Source: CAD feature listing. Evaluate the final solid. Frame: model axes, mm. A direction names the side the tool comes from. Round coordinates to 2 decimals unless told otherwise and drop trailing zeros. Order: outer loops, then holes, each group sorted by start corner. A loop starts at its lowest first (then second) coordinate and runs counter-clockwise, first axis right, second up. Notation, with made-up numbers: (6.5, 6.5) - (62.5, 6.5) arc R18 cw to (62.5, 13.5) - close; hole circle Ø10 at (33, 72.25). An arc over 180 degrees is marked (long way). Return JSON: item names as keys, results as strings. Group by question number.
1) Section A-A, the plane y = 8. Return loops of the section in (x, z).
2) Mould query, pull axis Z, two halves, no side actions, for faces 1 (the flat face through (4, 12.223, 7)), 2 (the cylindrical face through (-13.7, -10.8, 14.4)), 3 (the cylindrical face through (25.8, 9.7, 8)). Classes: pulls with the +Z half, pulls with the -Z half, needs draft (parallel to the pull), parting line crosses it, or undercut.
3) Ray query, line 1 (Y direction, x = -5, z = 4); line 2 (X direction, y = -20, z = 3); line 3 (Y direction, x = 25, z = 12.5). Return the intervals inside material, ascending. Write a range as from..to.
4) Section D-D, the plane y = -4.5. Return loops of the section in (x, z), plus the area to 3 significant figures.
5) Access query for faces 4 (the cylindrical face through (20.126, -8.102, 0.57)), 5 (the flat face through (3, -20.777, 4)), 6 (the cylindrical face through (20.126, -10.36, 14.43)), 7 (the cylindrical face through (22.13, 5.7, 9.43)). Directions: +Z, -Z, +X, -X, +Y, -Y. A direction counts if a zero-diameter tool reaches every point of the face in a straight line with its end or side. Return the directions, or none.
6) Contact query for flat-ended pins moving along their axis: P1, Ø8, axis at y = -8, z = 10, coming from the +X side; P2, Ø2.5, axis at x = 24.23, z = 7.5, coming from the +Y side; P3, Ø4, axis at y = -12.5, z = 5, coming from the -X side. Output: stop coordinate, or through.
7) Section C-C, the plane z = 7.5. Give the number of separate pieces and of enclosed holes in the cut face, plus the area to 3 significant figures.
8) Section B-B, the plane x = 25. Return loops of the section in (y, z).
```python
from build123d import *

# Parameters (mm, degrees)
F0_W     = 35
F0_H     = 25
F0_H_2   = 1.58
F0_H_3   = 5
F1_DEPTH = 15
F3_DEPTH = 9
F4_R     = 2
F6_SIZE  = 2
F5_R     = 1.65
F7_R     = 1.65
F8_DEPTH = 8.0000008897
F5_R_2   = 2.85
F7_R_2   = 2.85
F9_DEPTH = 3


with BuildPart() as f1:
    # F0 (on Top) → F1 (new body)
    with BuildSketch(Plane.XY):
        Polygon((28.2275901735, 12.2229893546), (-21.7724098265, 12.2229893546), (-21.7724098265, 4.2229884648), (-14.2724098265, 4.2229884648), (20.7275901735, 4.2229884648), (28.2275901735, 4.2229884648), align=None)
        with Locations((3.2275901735, -8.2770115352)):
            Rectangle(F0_W, F0_H)
        with Locations((3.2275901735, -21.5670115352)):
            Rectangle(F0_W, F0_H_2)
        with Locations((3.2275901735, -24.8570115352)):
            Rectangle(F0_W, F0_H_3)
    extrude(amount=F1_DEPTH)

    # F2 (on face) → F3 (cut)
    with BuildSketch(Plane.XY):
        with BuildLine():
            Line((19.5775901735, -21.6070115352), (19.8775901735, -21.6070115352))
            ThreePointArc((19.8775901735, -21.6070115352), (20.195788225, -21.7388134836), (20.3275901735, -22.0570115352))
            Line((20.3275901735, -22.0570115352), (20.3275901735, -22.3570115352))
            Line((20.3275901735, -22.3570115352), (20.7275901735, -22.3570115352))
            Line((20.7275901735, -22.3570115352), (20.7275901735, -20.7770115352))
            Line((20.7275901735, -20.7770115352), (-14.2724098265, -20.7770115352))
            Line((-14.2724098265, -20.7770115352), (-14.2724098265, -22.3570115352))
            Line((-14.2724098265, -22.3570115352), (-14.1524098265, -22.3570115352))
            Line((-14.1524098265, -22.3570115352), (-14.1524098265, -22.0570115352))
            ThreePointArc((-14.1524098265, -22.0570115352), (-14.0206078781, -21.7388134836), (-13.7024098265, -21.6070115352))
            Line((-13.7024098265, -21.6070115352), (-13.6128300801, -21.6070115352))
            Line((-13.6128300801, -21.6070115352), (-13.4024098265, -21.6070115352))
            ThreePointArc((-13.4024098265, -21.6070115352), (-13.084211775, -21.7388134836), (-12.9524098265, -22.0570115352))
            Line((-12.9524098265, -22.0570115352), (-12.9524098265, -22.3570115352))
            Line((-12.9524098265, -22.3570115352), (-12.0724098265, -22.3570115352))
            Line((-12.0724098265, -22.3570115352), (-12.0724098265, -22.0570115352))
            ThreePointArc((-12.0724098265, -22.0570115352), (-11.9406078781, -21.7388134836), (-11.6224098265, -21.6070115352))
            Line((-11.6224098265, -21.6070115352), (-11.3224098265, -21.6070115352))
            ThreePointArc((-11.3224098265, -21.6070115352), (-11.004211775, -21.7388134836), (-10.8724098265, -22.0570115352))
            Line((-10.8724098265, -22.0570115352), (-10.8724098265, -22.3570115352))
            Line((-10.8724098265, -22.3570115352), (-9.9924098265, -22.3570115352))
            Line((-9.9924098265, -22.3570115352), (-9.9924098265, -22.0570115352))
            ThreePointArc((-9.9924098265, -22.0570115352), (-9.8606078781, -21.7388134836), (-9.5424098265, -21.6070115352))
            Line((-9.5424098265, -21.6070115352), (-9.2424098265, -21.6070115352))
            ThreePointArc((-9.2424098265, -21.6070115352), (-8.924211775, -21.7388134836), (-8.7924098265, -22.0570115352))
            Line((-8.7924098265, -22.0570115352), (-8.7924098265, -22.3570115352))
            Line((-8.7924098265, -22.3570115352), (-7.9124098265, -22.3570115352))
            Line((-7.9124098265, -22.3570115352), (-7.9124098265, -22.0570115352))
            ThreePointArc((-7.9124098265, -22.0570115352), (-7.7806078781, -21.7388134836), (-7.4624098265, -21.6070115352))
            Line((-7.4624098265, -21.6070115352), (-7.1624098265, -21.6070115352))
            ThreePointArc((-7.1624098265, -21.6070115352), (-6.844211775, -21.7388134836), (-6.7124098265, -22.0570115352))
            Line((-6.7124098265, -22.0570115352), (-6.7124098265, -22.3570115352))
            Line((-6.7124098265, -22.3570115352), (-5.8324098265, -22.3570115352))
            Line((-5.8324098265, -22.3570115352), (-5.8324098265, -22.0570115352))
            ThreePointArc((-5.8324098265, -22.0570115352), (-5.7006078781, -21.7388134836), (-5.3824098265, -21.6070115352))
            Line((-5.3824098265, -21.6070115352), (-5.0824098265, -21.6070115352))
            ThreePointArc((-5.0824098265, -21.6070115352), (-4.764211775, -21.7388134836), (-4.6324098265, -22.0570115352))
            Line((-4.6324098265, -22.0570115352), (-4.6324098265, -22.3570115352))
            Line((-4.6324098265, -22.3570115352), (-3.7524098265, -22.3570115352))
            Line((-3.7524098265, -22.3570115352), (-3.7524098265, -22.0570115352))
            ThreePointArc((-3.7524098265, -22.0570115352), (-3.6206078781, -21.7388134836), (-3.3024098265, -21.6070115352))
            Line((-3.3024098265, -21.6070115352), (-3.0024098265, -21.6070115352))
            ThreePointArc((-3.0024098265, -21.6070115352), (-2.684211775, -21.7388134836), (-2.5524098265, -22.0570115352))
            Line((-2.5524098265, -22.0570115352), (-2.5524098265, -22.3570115352))
            Line((-2.5524098265, -22.3570115352), (-1.6724098265, -22.3570115352))
            Line((-1.6724098265, -22.3570115352), (-1.6724098265, -22.0570115352))
            ThreePointArc((-1.6724098265, -22.0570115352), (-1.5406078781, -21.7388134836), (-1.2224098265, -21.6070115352))
            Line((-1.2224098265, -21.6070115352), (-0.9224098265, -21.6070115352))
            ThreePointArc((-0.9224098265, -21.6070115352), (-0.604211775, -21.7388134836), (-0.4724098265, -22.0570115352))
            Line((-0.4724098265, -22.0570115352), (-0.4724098265, -22.3570115352))
            Line((-0.4724098265, -22.3570115352), (0.4075901735, -22.3570115352))
            Line((0.4075901735, -22.3570115352), (0.4075901735, -22.0570115352))
            ThreePointArc((0.4075901735, -22.0570115352), (0.5393921219, -21.7388134836), (0.8575901735, -21.6070115352))
            Line((0.8575901735, -21.6070115352), (1.1575901735, -21.6070115352))
            ThreePointArc((1.1575901735, -21.6070115352), (1.475788225, -21.7388134836), (1.6075901735, -22.0570115352))
            Line((1.6075901735, -22.0570115352), (1.6075901735, -22.3570115352))
            Line((1.6075901735, -22.3570115352), (2.4875901735, -22.3570115352))
            Line((2.4875901735, -22.3570115352), (2.4875901735, -22.0570115352))
            ThreePointArc((2.4875901735, -22.0570115352), (2.6193921219, -21.7388134836), (2.9375901735, -21.6070115352))
            Line((2.9375901735, -21.6070115352), (3.2375901735, -21.6070115352))
            ThreePointArc((3.2375901735, -21.6070115352), (3.555788225, -21.7388134836), (3.6875901735, -22.0570115352))
            Line((3.6875901735, -22.0570115352), (3.6875901735, -22.3570115352))
            Line((3.6875901735, -22.3570115352), (4.5675901735, -22.3570115352))
            Line((4.5675901735, -22.3570115352), (4.5675901735, -22.0570115352))
            ThreePointArc((4.5675901735, -22.0570115352), (4.6993921219, -21.7388134836), (5.0175901735, -21.6070115352))
            Line((5.0175901735, -21.6070115352), (5.3175901735, -21.6070115352))
            ThreePointArc((5.3175901735, -21.6070115352), (5.635788225, -21.7388134836), (5.7675901735, -22.0570115352))
            Line((5.7675901735, -22.0570115352), (5.7675901735, -22.3570115352))
            Line((5.7675901735, -22.3570115352), (6.6475901735, -22.3570115352))
            Line((6.6475901735, -22.3570115352), (6.6475901735, -22.0570115352))
            ThreePointArc((6.6475901735, -22.0570115352), (6.7793921219, -21.7388134836), (7.0975901735, -21.6070115352))
            Line((7.0975901735, -21.6070115352), (7.3975901735, -21.6070115352))
            ThreePointArc((7.3975901735, -21.6070115352), (7.715788225, -21.7388134836), (7.8475901735, -22.0570115352))
            Line((7.8475901735, -22.0570115352), (7.8475901735, -22.3570115352))
            Line((7.8475901735, -22.3570115352), (8.7275901735, -22.3570115352))
            Line((8.7275901735, -22.3570115352), (8.7275901735, -22.0570115352))
            ThreePointArc((8.7275901735, -22.0570115352), (8.8593921219, -21.7388134836), (9.1775901735, -21.6070115352))
            Line((9.1775901735, -21.6070115352), (9.4775901735, -21.6070115352))
            ThreePointArc((9.4775901735, -21.6070115352), (9.795788225, -21.7388134836), (9.9275901735, -22.0570115352))
            Line((9.9275901735, -22.0570115352), (9.9275901735, -22.3570115352))
            Line((9.9275901735, -22.3570115352), (10.8075901735, -22.3570115352))
            Line((10.8075901735, -22.3570115352), (10.8075901735, -22.0570115352))
            ThreePointArc((10.8075901735, -22.0570115352), (10.9393921219, -21.7388134836), (11.2575901735, -21.6070115352))
            Line((11.2575901735, -21.6070115352), (11.5575901735, -21.6070115352))
            ThreePointArc((11.5575901735, -21.6070115352), (11.875788225, -21.7388134836), (12.0075901735, -22.0570115352))
            Line((12.0075901735, -22.0570115352), (12.0075901735, -22.3570115352))
            Line((12.0075901735, -22.3570115352), (12.8875901735, -22.3570115352))
            Line((12.8875901735, -22.3570115352), (12.8875901735, -22.0570115352))
            ThreePointArc((12.8875901735, -22.0570115352), (13.0193921219, -21.7388134836), (13.3375901735, -21.6070115352))
            Line((13.3375901735, -21.6070115352), (13.6375901735, -21.6070115352))
            ThreePointArc((13.6375901735, -21.6070115352), (13.955788225, -21.7388134836), (14.0875901735, -22.0570115352))
            Line((14.0875901735, -22.0570115352), (14.0875901735, -22.3570115352))
            Line((14.0875901735, -22.3570115352), (14.9675901735, -22.3570115352))
            Line((14.9675901735, -22.3570115352), (14.9675901735, -22.0570115352))
            ThreePointArc((14.9675901735, -22.0570115352), (15.0993921219, -21.7388134836), (15.4175901735, -21.6070115352))
            Line((15.4175901735, -21.6070115352), (15.7175901735, -21.6070115352))
            ThreePointArc((15.7175901735, -21.6070115352), (16.035788225, -21.7388134836), (16.1675901735, -22.0570115352))
            Line((16.1675901735, -22.0570115352), (16.1675901735, -22.3570115352))
            Line((16.1675901735, -22.3570115352), (17.0475901735, -22.3570115352))
            Line((17.0475901735, -22.3570115352), (17.0475901735, -22.0570115352))
            ThreePointArc((17.0475901735, -22.0570115352), (17.1793921219, -21.7388134836), (17.4975901735, -21.6070115352))
            Line((17.4975901735, -21.6070115352), (17.7975901735, -21.6070115352))
            ThreePointArc((17.7975901735, -21.6070115352), (18.115788225, -21.7388134836), (18.2475901735, -22.0570115352))
            Line((18.2475901735, -22.0570115352), (18.2475901735, -22.3570115352))
            Line((18.2475901735, -22.3570115352), (19.1275901735, -22.3570115352))
            Line((19.1275901735, -22.3570115352), (19.1275901735, -22.0570115352))
            ThreePointArc((19.1275901735, -22.0570115352), (19.2593921219, -21.7388134836), (19.5775901735, -21.6070115352))
        make_face()
    extrude(amount=F3_DEPTH, mode=Mode.SUBTRACT)

    # F4
    f4_edges = [f1.edges().sort_by_distance(p)[0] for p in [
        (-14.27241, -8.277012, 0),
        (-14.27241, -11.567012, 15),
        (20.72759, -11.567012, 15),
        (20.72759, -8.277012, 0),
        (3.22759, -27.357012, 0),
        (3.22759, -27.357012, 15),
        (20.72759, -27.357012, 7.5),
        (-14.27241, -27.357012, 7.5),
        (20.72759, -24.857012, 0),
        (-14.27241, -24.857012, 0),
    ]]
    fillet(f4_edges, radius=F4_R)

    # F6
    f6_edges = [f1.edges().sort_by_distance(p)[0] for p in [
        (-21.77241, 8.222989, 0),
        (-21.77241, 8.222989, 15),
        (28.22759, 8.222989, 0),
        (28.22759, 8.222989, 15),
    ]]
    chamfer(f6_edges, length=F6_SIZE)

    # F5 (on face) + F7 (on face) → F8 (cut, through all)
    with BuildSketch(Plane.XZ.offset(-4.2229884648)):
        with Locations((24.2275901735, 7.5)):
            Circle(F5_R)
    with BuildSketch(Plane.XZ.offset(-4.2229884648)):
        with Locations((-17.7724098265, 7.5)):
            Circle(F7_R)
    extrude(amount=-F8_DEPTH, mode=Mode.SUBTRACT)

    # F5 (on face) + F7 (on face) → F9 (cut)
    with BuildSketch(Plane.XZ.offset(-4.2229884648)):
        with Locations((24.2275901735, 7.5)):
            Circle(F5_R_2)
        with Locations((24.2275901735, 7.5)):
            Circle(F5_R, mode=Mode.SUBTRACT)
    with BuildSketch(Plane.XZ.offset(-4.2229884648)):
        with Locations((-17.7724098265, 7.5)):
            Circle(F7_R_2)
        with Locations((-17.7724098265, 7.5)):
            Circle(F7_R, mode=Mode.SUBTRACT)
    extrude(amount=-F9_DEPTH, mode=Mode.SUBTRACT)


solid = f1.part
```
Geometry check:
{
 "1": {"outline": "(-21.77, 2) - (-19.77, 0) - (26.23, 0) - (28.23, 2) - (28.23, 13) - (26.23, 15) - (-19.77, 15) - (-21.77, 13) - close; hole circle Ø3.3 at (-17.77, 7.5); hole circle Ø3.3 at (24.23, 7.5)"},
 "2": {"face 1": "needs draft", "face 2": "pulls with the +Z half", "face 3": "undercut"},
 "3": {"line 1": "-27.36..-21.61, -20.78..12.22", "line 2": "-14.27..20.73", "line 3": "4.22..12.22"},
 "4": {"outline": "(-14.27, 2) arc R2 ccw to (-12.27, 0) - (18.73, 0) arc R2 ccw to (20.73, 2) - (20.73, 13) arc R2 ccw to (18.73, 15) - (-12.27, 15) arc R2 ccw to (-14.27, 13) - close", "area": "522 mm2"},
 "5": {"face 4": "-Z, +X, -Y", "face 5": "-Z, +X, -X", "face 6": "+Z, +X, -Y", "face 7": "-Y"},
 "6": {"P1": "x = 20.73", "P2": "through", "P3": "x = -14.27"},
 "7": {"separate pieces": "4", "enclosed holes": "0", "area": "1,390 mm2"},
 "8": {"outline": "(4.22, 0) - (12.22, 0) - (12.22, 6.04) - (7.22, 6.04) - (7.22, 4.76) - (4.22, 4.76) - close; (4.22, 10.24) - (7.22, 10.24) - (7.22, 8.96) - (12.22, 8.96) - (12.22, 15) - (4.22, 15) - close"}
}
